```python
from build123d import *

# Parameters (mm, degrees)
SKETCH1_R           = 3.98
BOSS_EXTRUDE1_DEPTH = 6
FILLET1_R           = 0.35
CHAMFER1_SIZE       = 1.5


with BuildPart() as part:
    # Sketch1 → Boss-Extrude1 (new body)
    with BuildSketch(Plane(origin=(0, 0, 0), x_dir=(1, 0, 0), z_dir=(0, 1, 0))):
        with BuildLine():
            Line((-14.732151132, 3), (-22.015934783, 3))
            ThreePointArc((-22.015934783, 3), (-39.46, 0), (-22.015934783, -3))
            Line((-22.015934783, -3), (-5.802039289, -3))
            Line((-5.802039289, -3), (-6.876644452, -4.996174644))
            Line((-6.876644452, -4.996174644), (-4.608220474, -4.58413613))
            ThreePointArc((-4.608220474, -4.58413613), (-4.596194078, -4.596194078), (-4.58413613, -4.608220474))
            Line((-4.58413613, -4.608220474), (-4.996174644, -6.876644452))
            Line((-4.996174644, -6.876644452), (-2.966102142, -5.783790979))
            ThreePointArc((-2.966102142, -5.783790979), (-2.950938248, -5.791542407), (-2.935754098, -5.799254079))
            Line((-2.935754098, -5.799254079), (-2.626644452, -8.083980389))
            Line((-2.626644452, -8.083980389), (-1.033641065, -6.417288068))
            ThreePointArc((-1.033641065, -6.417288068), (-1.016824023, -6.419974214), (-1, -6.422616289))
            Line((-1, -6.422616289), (0, -8.5))
            Line((0, -8.5), (1, -6.422616289))
            ThreePointArc((1, -6.422616289), (1.016824023, -6.419974214), (1.033641065, -6.417288068))
            Line((1.033641065, -6.417288068), (2.626644452, -8.083980389))
            Line((2.626644452, -8.083980389), (2.935754098, -5.799254079))
            ThreePointArc((2.935754098, -5.799254079), (2.950938248, -5.791542407), (2.966102142, -5.783790979))
            Line((2.966102142, -5.783790979), (4.996174644, -6.876644452))
            Line((4.996174644, -6.876644452), (4.58413613, -4.608220474))
            ThreePointArc((4.58413613, -4.608220474), (4.596194078, -4.596194078), (4.608220474, -4.58413613))
            Line((4.608220474, -4.58413613), (6.876644452, -4.996174644))
            Line((6.876644452, -4.996174644), (5.783790979, -2.966102142))
            ThreePointArc((5.783790979, -2.966102142), (5.791542407, -2.950938248), (5.799254079, -2.935754098))
            Line((5.799254079, -2.935754098), (8.083980389, -2.626644452))
            Line((8.083980389, -2.626644452), (6.417288068, -1.033641065))
            ThreePointArc((6.417288068, -1.033641065), (6.419974214, -1.016824023), (6.422616289, -1))
            Line((6.422616289, -1), (8.5, 0))
            Line((8.5, 0), (6.422616289, 1))
            ThreePointArc((6.422616289, 1), (6.419974214, 1.016824023), (6.417288068, 1.033641065))
            Line((6.417288068, 1.033641065), (8.083980389, 2.626644452))
            Line((8.083980389, 2.626644452), (5.799254079, 2.935754098))
            ThreePointArc((5.799254079, 2.935754098), (5.791542407, 2.950938248), (5.783790979, 2.966102142))
            Line((5.783790979, 2.966102142), (6.876644452, 4.996174644))
            Line((6.876644452, 4.996174644), (4.608220474, 4.58413613))
            ThreePointArc((4.608220474, 4.58413613), (4.596194078, 4.596194078), (4.58413613, 4.608220474))
            Line((4.58413613, 4.608220474), (4.996174644, 6.876644452))
            Line((4.996174644, 6.876644452), (2.966102142, 5.783790979))
            ThreePointArc((2.966102142, 5.783790979), (2.950938248, 5.791542407), (2.935754098, 5.799254079))
            Line((2.935754098, 5.799254079), (2.626644452, 8.083980389))
            Line((2.626644452, 8.083980389), (1.033641065, 6.417288068))
            ThreePointArc((1.033641065, 6.417288068), (1.016824023, 6.419974214), (1, 6.422616289))
            Line((1, 6.422616289), (0, 8.5))
            Line((0, 8.5), (-1, 6.422616289))
            ThreePointArc((-1, 6.422616289), (-1.016824023, 6.419974214), (-1.033641065, 6.417288068))
            Line((-1.033641065, 6.417288068), (-2.626644452, 8.083980389))
            Line((-2.626644452, 8.083980389), (-2.935754098, 5.799254079))
            ThreePointArc((-2.935754098, 5.799254079), (-2.950938248, 5.791542407), (-2.966102142, 5.783790979))
            Line((-2.966102142, 5.783790979), (-4.996174644, 6.876644452))
            Line((-4.996174644, 6.876644452), (-4.58413613, 4.608220474))
            ThreePointArc((-4.58413613, 4.608220474), (-4.596194078, 4.596194078), (-4.608220474, 4.58413613))
            Line((-4.608220474, 4.58413613), (-6.876644452, 4.996174644))
            Line((-6.876644452, 4.996174644), (-5.802039289, 3))
            Line((-5.802039289, 3), (-14.732151132, 3))
        make_face()
        with Locations(Location((-30.48, 0, 0), (0, 0, 270))):
            Circle(SKETCH1_R, mode=Mode.SUBTRACT)
        with Locations(Location((0, 0, 0), (0, 0, 270))):
            Circle(SKETCH1_R, mode=Mode.SUBTRACT)
    extrude(amount=BOSS_EXTRUDE1_DEPTH)

    # Fillet1
    fillet1_edges = [part.edges().sort_by_distance(p)[0] for p in [
        (0, 3, 8.5),
        (-2.626644452, 3, 8.083980389),
        (-4.996174644, 3, 6.876644452),
        (-6.876644452, 3, 4.996174644),
        (-6.876644452, 3, -4.996174644),
        (-4.996174644, 3, -6.876644452),
        (-2.626644452, 3, -8.083980389),
        (0, 3, -8.5),
        (2.626644452, 3, -8.083980389),
        (4.996174644, 3, -6.876644452),
        (6.876644452, 3, -4.996174644),
        (8.083980389, 3, -2.626644452),
        (8.5, 3, 0),
        (8.083980389, 3, 2.626644452),
        (6.876644452, 3, 4.996174644),
        (4.996174644, 3, 6.876644452),
        (2.626644452, 3, 8.083980389),
    ]]
    fillet(fillet1_edges, radius=FILLET1_R)

    # Chamfer1
    chamfer1_edges = [part.edges().sort_by_distance(p)[0] for p in [
        (-13.908987036, 6, -3),
        (-39.46, 6, 0),
        (-13.908987036, 6, 3),
        (-13.908987036, 0, 3),
        (-39.46, 0, 0),
        (-13.908987036, 0, -3),
    ]]
    chamfer(chamfer1_edges, length=CHAMFER1_SIZE)


solid = part.part
```
Read the model definition and answer for the solid it produces. Units are mm, in the model's axes. A direction names the side the tool comes from. Round coordinates to 2 decimals unless told otherwise and drop trailing zeros. Write each loop counter-clockwise with the first axis right and the second up, starting at its lowest first coordinate (ties: lowest second). Pieces come first, ordered by that corner, then holes. Notation, with made-up numbers: M -14.75,-34 L 11.25,-34 A21 ccw 11.25,-17 Z; hole C 0.25,8.5 d2. An arc over 180 degrees is marked long. One line per item, written item: value.
Q1. Flat-ended cylindrical pins translate along their axes: pin 1 Ø1.5 at (y, z) = (5, -1.5) entering from -X; pin 2 Ø10.5 at (x, z) = (-30.48, 0) entering from -Y; pin 3 Ø2.5 at (x, y) = (-14, 2.5) entering from +Z; pin 4 Ø2.5 at (x, y) = (-11, 2.5) entering from -Z. Find the tip coordinate at first contact, or state that the pin passes through.
Data:
pin 1: x = -39.41
pin 2: y = 0
pin 3: z = 3
pin 4: z = -3
Q2. For a pull along Z with two mould halves and no side action, classify faces 1 (the flat face through (7.124, 2.958, 0.662)), 2 (the flat face through (4.723, 2.958, -5.374)), 3 (the flat face through (1.57, 2.96, 6.98)), 4 (the flat face through (-15, 0, 0)) as +Z half, -Z half, draft (parallel to the pull), parting line (faces both ways), or undercut.
Data:
face 1: undercut
face 2: undercut
face 3: +Z half
face 4: draft
Q3. Find section A-A on x = -30.48. Write down the section's boundary in (y, z), plus the area to 3 significant figures.
Data:
outline: M 0,-7.48 L 1.5,-8.98 L 4.5,-8.98 L 6,-7.48 L 6,-3.98 L 0,-3.98 Z; M 0,3.98 L 6,3.98 L 6,7.48 L 4.5,8.98 L 1.5,8.98 L 0,7.48 Z
area: 55.5 mm2
Q4. Find section C-C on z = 3.5. Count the separate pieces of the cut face and the enclosed holes in it, plus the area to 3 significant figures.
Data:
separate pieces: 4
enclosed holes: 0
area: 122 mm2
Q5. Which of the six approach directions +Z, -Z, +X, -X, +Y, -Y give full straight-line access (tool end or side, diameter ignored) to faces 5 (the flat face through (3.671, 2.958, -6.163)), 6 (the flat face through (6.59, 2.96, -2.83)), 7 (the flat face through (-15, 6, 0)), 8 (the flat face through (-1.59, 2.96, 7))?
Data:
face 5: -Z, +Y, -Y
face 6: +X, +Y, -Y
face 7: +Z, -Z, +X, -X, +Y
face 8: +Z, +Y, -Y
Q6. Find section B-B on x = -19.5. Write down the section's boundary in (y, z).
Data:
outline: M 0,-1.5 L 1.5,-3 L 4.5,-3 L 6,-1.5 L 6,1.5 L 4.5,3 L 1.5,3 L 0,1.5 Z
Q7. Straight lines are drawn through the part: line 1 (X direction, y = 2.45, z = 0); line 2 (Z direction, x = -19, y = 2.5); line 3 (X direction, y = 0.5, z = 0.5). For each, find the intervals that lie inside material, in ascending order. Write a range as [from, to].
Data:
line 1: [-39.46, -34.46], [-26.5, -3.98], [3.98, 8.04]
line 2: [-3, 3]
line 3: [-38.44, -34.43], [-26.53, -3.95], [3.95, 7.46]
